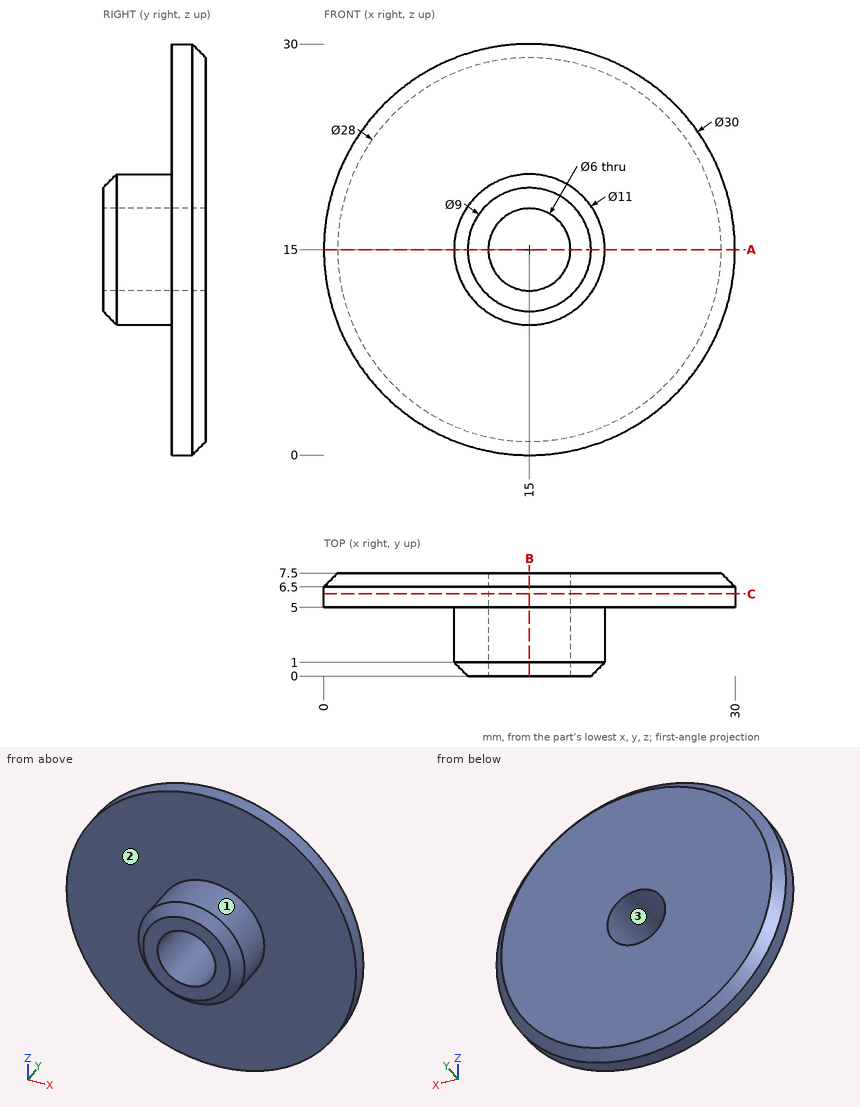
Source: three-view drawing plus pictorial views. Frame: mm from the lowest corner of the part. Round coordinates to 2 decimals unless told otherwise and drop trailing zeros. Order: outer loops, then holes, each group sorted by start corner. A loop starts at its lowest first (then second) coordinate and runs counter-clockwise, first axis right, second up. Notation, with made-up numbers: (25, 43.25) -> (31, 43.25) arc R31 ccw to (31, 75.25) -> close; hole circle Ø1 at (14.5, 22). An arc over 180 degrees is marked (long way). Use CSV: the item, a comma, the result in double quotes. Start each with the question number.
1) Section A-A (z = 15). Return the cut outline in (x, y), and give its area (3 significant figures).
2) Draft query along Z for the marked faces 1, 2 and 3. Return one class per face: +Z half, -Z half, draft (parallel to the pull), parting line (faces both ways), or undercut.
3) Section B-B (x = 15). Return the cut outline in (y, z), and give its area (3 significant figures).
4) First-contact query: pin 1 Ø1.5 at (x, y) = (17.5, 4) entering from -Z; pin 2 Ø3 at (y, z) = (6.5, 23.5) entering from +X; pin 3 Ø3 at (x, y) = (5, 2) entering from -Z. Flat tips, straight axial feed; report the tip coordinate or a pass-through.
5) Material intervals for line 1 along Z through (x, y) = (15, 2.75); line 2 along Z through (x, y) = (15, 5.25); line 3 along Y through (x, z) = (7.25, 10), sorted ascending. Write a range as from..to.
6) Section C-C (y = 6). Return the cut outline in (x, z), and give its area (3 significant figures).
Returned:
1,outline,"(0, 5) -> (9.5, 5) -> (9.5, 1) -> (10.5, 0) -> (12, 0) -> (12, 7.5) -> (1, 7.5) -> (0, 6.5) -> close; (18, 0) -> (19.5, 0) -> (20.5, 1) -> (20.5, 5) -> (30, 5) -> (30, 6.5) -> (29, 7.5) -> (18, 7.5) -> close"
1,area,"83.0 mm²"
2,face 1,"parting line"
2,face 2,"draft"
2,face 3,"undercut"
3,outline,"(0, 10.5) -> (1, 9.5) -> (5, 9.5) -> (5, 0) -> (6.5, 0) -> (7.5, 1) -> (7.5, 12) -> (0, 12) -> close; (0, 18) -> (7.5, 18) -> (7.5, 29) -> (6.5, 30) -> (5, 30) -> (5, 20.5) -> (1, 20.5) -> (0, 19.5) -> close"
3,area,"83.0 mm²"
4,pin 1,"stops at z = 9.79"
4,pin 2,"stops at x = 28.27"
4,pin 3,"passes through"
5,line 1,"z = 9.5..12, 18..20.5"
5,line 2,"z = 0..12, 18..30"
5,line 3,"y = 5..7.5"
6,outline,"circle Ø30 at (15, 15); hole circle Ø6 at (15, 15)"
6,area,"679 mm²"
